Geometry: final body of the model. Coordinates: model frame, mm. Round coordinates to 2 decimals unless told otherwise and drop trailing zeros. Order: outer loops, then holes, each group sorted by start corner. A loop starts at its lowest first (then second) coordinate and runs counter-clockwise, first axis right, second up. Notation, with made-up numbers: (88, 66.25) - (142, 66.25) arc R20 cw to (142, 78.25) - close; hole circle Ø7 at (35, 22). An arc over 180 degrees is marked (long way). Put each result on its own line as item: value. Start each with the question number.
(1) Section C-C (x = 2.75). Output: boundary loops of the cut face in (y, z), and give its area (3 significant figures).
(2) Section B-B (z = 0). Output: boundary loops of the cut face in (x, y).
(3) Section D-D (z = -2). Output: boundary loops of the cut face in (x, y).
(4) Section A-A (y = 0). Output: boundary loops of the cut face in (x, z).
(5) Pull-direction query (Y, two-part tool) for faces 1 (the face through (14.297, -1.949, 1.965)), 2 (the face through (14, 1, 2.25)), 3 (the face through (13.9, 0.27, -0.86)); classes: released by +Y, released by -Y, zero draft, split by the parting line, or undercut.
(6) Material intervals for L1, parallel to Y at x = 14.75, z = 0; L2, parallel to Y at x = 16.5, z = -1.75; L3, parallel to Y at x = 16.25, z = -0.5, sorted ascending. Write a range as [from, to].
(7) Pin query (flat end, axial travel): P1, Ø1.5, axis at x = 14.5, y = 0.5, coming from the -Z side; P2, Ø1.4, axis at y = 0, z = 0, coming from the -X side; P3, Ø2, axis at x = 4, y = 0, coming from the -Z side; P4, Ø1, axis at x = 7.5, z = -1, coming from the +Y side. Return the tip coordinate at first contact, or that it passes through.
from build123d import *

# Parameters (mm, degrees)
SKETCH1_R           = 0.9
BOSS_EXTRUDE1_DEPTH = 28.2
FILLET1_R           = 1


with BuildPart() as part:
    # Sketch1 → Boss-Extrude1 (new body)
    with BuildSketch(Plane(origin=(0, 0, 0), x_dir=(0, 0, -1), z_dir=(1, 0, 0))):
        Polygon((-2.25, 5.75), (-2.25, -2.25), (5.75, -2.25), align=None)
        Circle(SKETCH1_R, mode=Mode.SUBTRACT)
    extrude(amount=BOSS_EXTRUDE1_DEPTH)

    # Fillet1
    fillet1_edges = [part.edges().sort_by_distance(p)[0] for p in [
        (14.1, -2.25, -5.75),
        (14.1, -2.25, 2.25),
        (14.1, 5.75, 2.25),
    ]]
    fillet(fillet1_edges, radius=FILLET1_R)


solid = part.part
Checks:
1. outline: (-2.25, -3.34) arc R1 ccw to (-0.54, -4.04) - (4.04, 0.54) arc R1 ccw to (3.34, 2.25) - (-1.25, 2.25) arc R1 ccw to (-2.25, 1.25) - close; hole circle Ø1.8 at (0, 0)
1. area: 26.8 mm²
2. outline: (0, -2.25) - (28.2, -2.25) - (28.2, -0.9) - (0, -0.9) - close; (0, 0.9) - (28.2, 0.9) - (28.2, 3.5) - (0, 3.5) - close
3. outline: (0, -2.25) - (28.2, -2.25) - (28.2, 1.5) - (0, 1.5) - close
4. outline: (0, -3.5) - (28.2, -3.5) - (28.2, -0.9) - (0, -0.9) - close; (0, 0.9) - (28.2, 0.9) - (28.2, 2.25) - (0, 2.25) - close
5. face 1: released by -Y
5. face 2: zero draft
5. face 3: undercut
6. L1: y = [-2.25, -0.9], [0.9, 3.5]
6. L2: y = [-2.25, 1.75]
6. L3: y = [-2.25, -0.75], [0.75, 3]
7. P1: stops at z = -3.75
7. P2: passes through
7. P3: stops at z = -4.3
7. P4: stops at y = 3
